For this review, take the finished solid that the model builds, in its own axes (mm). Face numbers are marked on the shaded views. A direction names the side the tool comes from. Give positions to 0.01 mm unless a question says otherwise; leave off trailing zeros. Loops run counter-clockwise (first coordinate to the right, second up) from the corner with the lowest first, then second, coordinate; pieces in that order, holes last. Notation, with made-up numbers: M 83.25,-35.75 L 138.25,-35.75 A17 cw 138.25,-7.75 Z; hole C -4,69.25 d7. An arc over 180 degrees is marked long. Use CSV: the item, a comma, the result in double quotes. Start each with the question number.
1. Tool access review of the marked faces 4 and 5: name each direction out of +Z, -Z, +X, -X, +Y, -Y from which nothing blocks a thin tool from reaching the whole face with its end or side.
2. To check wall thickness, follow line 1 (X direction, y = 7.5, z = -5); line 2 (X direction, y = 20, z = 5); line 3 (X direction, y = 3.75, z = -6.5). State the ranges of each line that lie inside material, in increasing order. Write a range as [from, to].
3. Insertion check: P1, Ø4, axis at x = 6, z = -5, coming from the +Y side; P2, Ø5, axis at x = -27.5, z = 1, coming from the -Y side. Each pin has a flat end and moves straight along its axis. Give the tip position at first contact, or say it passes through.
4. The part is to be moulded in two halves that separate along Z. For the marked faces 1, 2 and 3, say which applies: pulls with the +Z half, pulls with the -Z half, needs draft (parallel to the pull), parting line crosses it, or undercut.
5. Take a section at D-D, the plane y = 18.5. Write out the cut boundary in (x, z).
6. Take a section at B-B, the plane z = 5. Write out the cut boundary in (x, y), and give its area (3 significant figures).
7. Take a section at A-A, the plane y = 5.5. Write out the cut boundary in (x, z), and give its area (3 significant figures).
8. Take a section at C-C, the plane x = -34. Write out the cut boundary in (y, z).
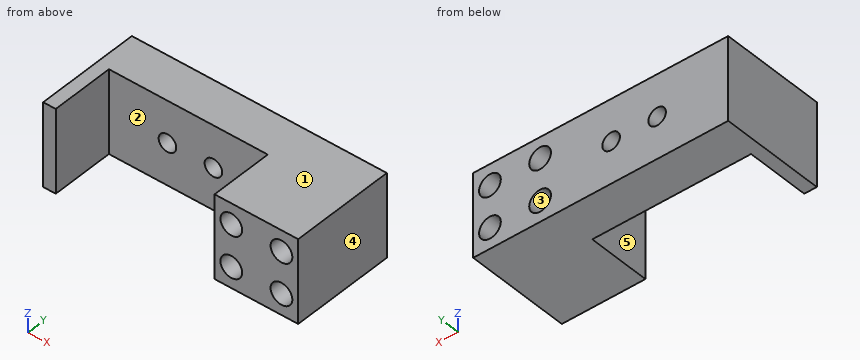
from build123d import *

# Parameters (mm, degrees)
SKETCH_1_W          = 20
SKETCH_1_H          = 20
SKETCH_1_R          = 2.6
EXTRUDE_1_DEPTH     = 25
SKETCH_2_W          = 41
SKETCH_2_H          = 20
EXTRUDE_2_DEPTH     = 10
SKETCH_3_W          = 3
SKETCH_3_H          = 20
EXTRUDE_3_DEPTH     = 15
SKETCH_4_R          = 2.1
CUT_EXTRUDE_1_DEPTH = 58.671483421


with BuildPart() as part:
    # 草图1 → 凸台-拉伸1 (new body)
    with BuildSketch(Plane(origin=(0, 0, 0), x_dir=(1, 0, 0), z_dir=(0, 1, 0))):
        Rectangle(SKETCH_1_W, SKETCH_1_H)
        with Locations(Location((-6, 5, 0), (0, 0, 270))):
            Circle(SKETCH_1_R, mode=Mode.SUBTRACT)
        with Locations(Location((6, 5, 0), (0, 0, 270))):
            Circle(SKETCH_1_R, mode=Mode.SUBTRACT)
        with Locations(Location((-6, -5, 0), (0, 0, 270))):
            Circle(SKETCH_1_R, mode=Mode.SUBTRACT)
        with Locations(Location((6, -5, 0), (0, 0, 270))):
            Circle(SKETCH_1_R, mode=Mode.SUBTRACT)
    extrude(amount=EXTRUDE_1_DEPTH)

    # 草图2 → 凸台-拉伸2 (add)
    with BuildSketch(Plane(origin=(0, 25, 0), x_dir=(1, 0, 0), z_dir=(0, 1, 0))):
        with Locations((-30.5, 0)):
            Rectangle(SKETCH_2_W, SKETCH_2_H)
    extrude(amount=-EXTRUDE_2_DEPTH)

    # 草图3 → 凸台-拉伸3 (add)
    with BuildSketch(Plane.XZ.offset(-15)):
        with Locations((-49.5, 0)):
            Rectangle(SKETCH_3_W, SKETCH_3_H)
    extrude(amount=EXTRUDE_3_DEPTH)

    # 草图4 → 切除-拉伸1 (cut, through all)
    with BuildSketch(Plane(origin=(0, 25, 0), x_dir=(1, 0, 0), z_dir=(0, 1, 0))):
        with Locations(Location((-34, 0, 0), (0, 0, 270))):
            Circle(SKETCH_4_R)
        with Locations(Location((-23, 0, 0), (0, 0, 270))):
            Circle(SKETCH_4_R)
    extrude(amount=-CUT_EXTRUDE_1_DEPTH, mode=Mode.SUBTRACT)


solid = part.part
Result set:
1,face 4,"+Z, -Z, +X, +Y, -Y"
1,face 5,"+Z, -Z, -Y"
2,line 1,"[-51, -48], [-10, -8.6], [-3.4, 3.4], [8.6, 10]"
2,line 2,"[-51, -8.6], [-3.4, 3.4], [8.6, 10]"
2,line 3,"[-51, -48], [-10, -8.12], [-3.88, 3.88], [8.12, 10]"
3,P1,"through"
3,P2,"y = 15"
4,face 1,"pulls with the +Z half"
4,face 2,"needs draft"
4,face 3,"undercut"
5,outline,"M -51,-10 L 10,-10 L 10,10 L -51,10 Z; hole C -34,0 d4.2; hole C -23,0 d4.2; hole C -6,-5 d5.2; hole C -6,5 d5.2; hole C 6,-5 d5.2; hole C 6,5 d5.2"
6,outline,"M -51,0 L -48,0 L -48,15 L -10,15 L -10,0 L -8.6,0 L -8.6,25 L -51,25 Z; M -3.4,0 L 3.4,0 L 3.4,25 L -3.4,25 Z; M 8.6,0 L 10,0 L 10,25 L 8.6,25 Z"
6,area,"695 mm2"
7,outline,"M -51,-10 L -48,-10 L -48,10 L -51,10 Z; M -10,-10 L 10,-10 L 10,10 L -10,10 Z; hole C -6,-5 d5.2; hole C -6,5 d5.2; hole C 6,-5 d5.2; hole C 6,5 d5.2"
7,area,"375 mm2"
8,outline,"M 15,-10 L 25,-10 L 25,-2.1 L 15,-2.1 Z; M 15,2.1 L 25,2.1 L 25,10 L 15,10 Z"
